```python
from build123d import *

# Parameters (mm, degrees)
SKETCH1_W                                  = 29
SKETCH1_H                                  = 6.5
TOP_PIECE_WITH_RIDGES_DEPTH                = 169
SUBTRACT_ACTUATOR_AND_BOTTOM_MOLD_OUTLIN_W = 3
SUBTRACT_ACTUATOR_AND_BOTTOM_MOLD_OUTLIN_H = 3
SUBTRACT_ACTUATOR_AND_BOTTOM_MOLD_DEPTH    = 169


# Read off the part's stored shape, not the designer's step: subtract actuator and bottom mold
with BuildPart() as part:
    # Sketch1 → top piece with ridges (new body)
    with BuildSketch(Plane(origin=(0, 0, 0), x_dir=(1, 0, 0), z_dir=(0, 1, 0))):
        with Locations((14.5, 3.25)):
            Rectangle(SKETCH1_W, SKETCH1_H)
    extrude(amount=TOP_PIECE_WITH_RIDGES_DEPTH)

    # subtract actuator and bottom mold outlin → subtract actuator and bottom mold (cut)
    with BuildSketch(Plane(origin=(0, 0, 0), x_dir=(1, 0, 0), z_dir=(0, 1, 0))):
        with Locations((27.5, 5)):
            Rectangle(SUBTRACT_ACTUATOR_AND_BOTTOM_MOLD_OUTLIN_W, SUBTRACT_ACTUATOR_AND_BOTTOM_MOLD_OUTLIN_H)
        with BuildLine():
            Line((23.85, 6.5), (5.15, 6.5))
            Line((5.15, 6.5), (5.15, 4.1))
            ThreePointArc((5.15, 4.1), (5.472182541, 3.322182541), (6.25, 3))
            Line((6.25, 3), (22.75, 3))
            ThreePointArc((22.75, 3), (23.527817459, 3.322182541), (23.85, 4.1))
            Line((23.85, 4.1), (23.85, 6.5))
        make_face()
        with Locations((1.5, 5)):
            Rectangle(SUBTRACT_ACTUATOR_AND_BOTTOM_MOLD_OUTLIN_W, SUBTRACT_ACTUATOR_AND_BOTTOM_MOLD_OUTLIN_H)
    extrude(amount=SUBTRACT_ACTUATOR_AND_BOTTOM_MOLD_DEPTH, mode=Mode.SUBTRACT)


solid = part.part
```
Verification items for the finished model (mm, model axes). A direction names the side the tool comes from. Round coordinates to 2 decimals unless told otherwise and drop trailing zeros. Write each loop counter-clockwise with the first axis right and the second up, starting at its lowest first coordinate (ties: lowest second). Pieces come first, ordered by that corner, then holes. Notation, with made-up numbers: (48, -19.75) - (73, -19.75) arc R16 cw to (73, -15.75) - close; hole circle Ø3 at (88.5, -15). An arc over 180 degrees is marked (long way). Answer as a JSON object with one key per item and string values. Group by question number.
Q1. Section check B-B, the plane y = 36. Enter the section's corners in (x, z).
Q2. Section check C-C, the plane x = 10.5. Enter the section's corners in (y, z), plus the area to 3 significant figures.
Q3. Go/stop test with flat-tipped pins: pin 1 Ø0.7 at (y, z) = (106, -5) entering from +X; pin 2 Ø1.5 at (x, y) = (1.5, 49.5) entering from -Z; pin 3 Ø0.7 at (y, z) = (78.5, -5.5) entering from -X. Record where each tip stops, or that it passes through.
Q4. Section check A-A, the plane z = -5.5. Enter the section's corners in (x, y), plus the area to 3 significant figures.
Q5. Tool access check on faces 1 (the flat face through (14, 83, -3)), 2 (the flat face through (3, 83, -5)), 3 (the flat face through (27, 83, -3.5)), 4 (the flat face through (29, 83, -2)). Record the directions out of +Z, -Z, +X, -X, +Y, -Y that give a thin tool (end or side, any length) a straight path to the whole face; none if there is none.
Q6. Thickness scan on line 1 (X direction, y = 141, z = -5.75); line 2 (Z direction, x = 6.75, y = 44); line 3 (Z direction, x = 5.5, y = 91). Record the ranges inside material, lowest first.
Found:
{
 "1": {"outline": "(0, -3.5) - (3, -3.5) - (3, -6.5) - (5.15, -6.5) - (5.15, -4.1) arc R1.1 cw to (6.25, -3) - (22.75, -3) arc R1.1 cw to (23.85, -4.1) - (23.85, -6.5) - (26, -6.5) - (26, -3.5) - (29, -3.5) - (29, 0) - (0, 0) - close"},
 "2": {"outline": "(0, -3) - (169, -3) - (169, 0) - (0, 0) - close", "area": "507 mm^2"},
 "3": {"pin 1": "stops at x = 26", "pin 2": "stops at z = -3.5", "pin 3": "stops at x = 3"},
 "4": {"outline": "(3, 0) - (5.15, 0) - (5.15, 169) - (3, 169) - close; (23.85, 0) - (26, 0) - (26, 169) - (23.85, 169) - close", "area": "727 mm^2"},
 "5": {"face 1": "-Z, +Y, -Y", "face 2": "-Z, -X, +Y, -Y", "face 3": "-Z, +X, +Y, -Y", "face 4": "+Z, -Z, +X, +Y, -Y"},
 "6": {"line 1": "x = 3 to 5.15, 23.85 to 26", "line 2": "z = -3 to 0", "line 3": "z = -3.3 to 0"}
}
